The listing builds one solid part. Answer for the finished solid, in the listing's coordinates (mm). Round coordinates to 2 decimals unless told otherwise and drop trailing zeros. Write each loop counter-clockwise with the first axis right and the second up, starting at its lowest first coordinate (ties: lowest second). Pieces come first, ordered by that corner, then holes. Notation, with made-up numbers: (21.25, 21.5) - (57.25, 21.5) arc R29 cw to (57.25, 45.5) - close; hole circle Ø10 at (52.5, 39). An arc over 180 degrees is marked (long way). Return JSON: item names as keys, results as strings. Group by question number.
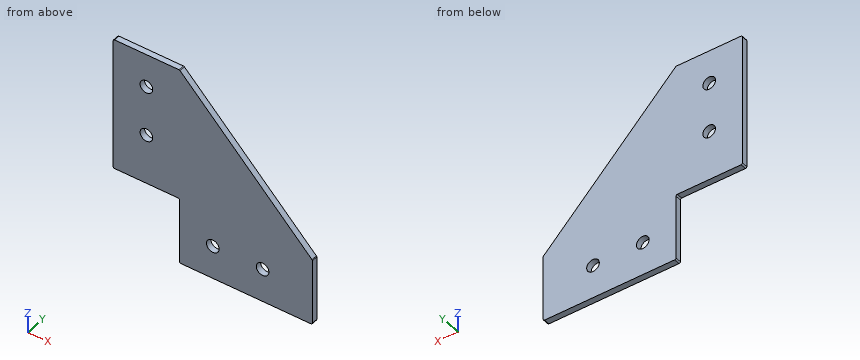
from build123d import *

# Parameters (mm, degrees)
F1_DEPTH = 2.286
F2_R     = 2.413
F3_DEPTH = 2.286
F4_R     = 0.508


with BuildPart() as f1:
    # F0 (on Front) → F1 (new body)
    with BuildSketch(Plane.XZ):
        Polygon((-14.859182, 44.231349), (-40.259182, 44.231349), (-40.259182, -6.568651), (-14.859182, -6.568651), (-14.859182, -31.968651), (35.940818, -31.968651), (35.940818, -6.568651), align=None)
    extrude(amount=F1_DEPTH)

    # F2 (on face) → F3 (cut)
    with BuildSketch(Plane.XZ.offset(2.286)):
        with Locations((-27.559182, 31.531349)):
            Circle(F2_R)
        with Locations((-27.559182, 12.481349)):
            Circle(F2_R)
        with Locations((-2.159182, -19.268651)):
            Circle(F2_R)
        with Locations((16.890818, -19.268651)):
            Circle(F2_R)
    extrude(amount=-F3_DEPTH, mode=Mode.SUBTRACT)

    # F4
    f4_edges = [f1.edges().sort_by_distance(p)[0] for p in [
        (-40.259182, -1.143, 44.231349),
        (-40.259182, -1.143, -6.568651),
        (-14.859182, -1.143, -31.968651),
        (-14.859182, -1.143, -6.568651),
        (35.940818, -1.143, -31.968651),
        (35.940818, -1.143, -6.568651),
        (-14.859182, -1.143, 44.231349),
    ]]
    fillet(f4_edges, radius=F4_R)


solid = f1.part
(1) Find section D-D (x = -21.5). Write down the section's boundary in (y, z), plus the area to 3 significant figures.
(2) Find section A-A (y = -1). Write down the section's boundary in (x, z).
(3) Find section B-B (x = -3.5). Write down the section's boundary in (y, z).
(4) Find section C-C (z = -26.5). Write down the section's boundary in (x, y), plus the area to 3 significant figures.
(5) Consider line 1 (X direction, y = -1.2, z = -19.5); line 2 (X direction, y = -1.4, z = -21); line 3 (X direction, y = -0.25, z = -8.5). Determine where each line is inside the solid, lowest interval first.
(6) Flat-ended cylindrical pins translate along their axes: pin 1 (4.5 mm diameter, centred on x = 16.89, z = -19.27, fed in from +Y); pin 2 (0.7 mm diameter, centred on y = -1, z = -14.5, fed in from -X); pin 3 (0.7 mm diameter, centred on x = -33.5, y = -1.5, fed in from -Z); pin 4 (1 mm diameter, centred on x = 19.5, y = -1, fed in from +Z). Find the tip coordinate at first contact, or state that the pin passes through.
Check sheet entries:
{
 "1": {"outline": "(-2.29, -6.57) - (0, -6.57) - (0, 44.23) - (-2.29, 44.23) - close", "area": "116 mm^2"},
 "2": {"outline": "(-40.26, -6.06) arc R0.51 ccw to (-39.75, -6.57) - (-15.37, -6.57) arc R0.51 cw to (-14.86, -7.08) - (-14.86, -31.46) arc R0.51 ccw to (-14.35, -31.97) - (35.43, -31.97) arc R0.51 ccw to (35.94, -31.46) - (35.94, -6.78) arc R0.51 ccw to (35.79, -6.42) - (-14.71, 44.08) arc R0.51 ccw to (-15.07, 44.23) - (-39.75, 44.23) arc R0.51 ccw to (-40.26, 43.72) - close; hole circle Ø4.83 at (-27.56, 12.48); hole circle Ø4.83 at (-27.56, 31.53); hole circle Ø4.83 at (-2.16, -19.27); hole circle Ø4.83 at (16.89, -19.27)"},
 "3": {"outline": "(-2.29, -31.97) - (0, -31.97) - (0, -21.27) - (-2.29, -21.27) - close; (-2.29, -17.26) - (0, -17.26) - (0, 32.87) - (-2.29, 32.87) - close"},
 "4": {"outline": "(-14.86, -2.29) - (35.94, -2.29) - (35.94, 0) - (-14.86, 0) - close", "area": "116 mm^2"},
 "5": {"line 1": "x = -14.86 to -4.56, 0.24 to 14.49, 19.29 to 35.94", "line 2": "x = -14.86 to -3.84, -0.48 to 15.21, 18.57 to 35.94", "line 3": "x = -14.86 to 35.94"},
 "6": {"pin 1": "passes through", "pin 2": "stops at x = -14.86", "pin 3": "stops at z = -6.57", "pin 4": "stops at z = 10.37"}
}
